Part model, mm, in its own coordinate system. A direction names the side the tool comes from. Coordinates: 2 decimals unless noted, no trailing zeros. Loops run counter-clockwise (first coordinate to the right, second up) from the corner with the lowest first, then second, coordinate; pieces in that order, holes last. Notation, with made-up numbers: M -33.75,47 L 2.25,47 A12 ccw 2.25,57 Z; hole C -8,38 d6. An arc over 180 degrees is marked long. Use a Markdown table: item, result. Add a question column.
1) Band-saw the part on D-D (z = 51). List the corners of the cut face in (x, y).
2) Band-saw the part on C-C (x = 0). List the corners of the cut face in (y, z).
3) Band-saw the part on A-A (x = 22.5). List the corners of the cut face in (y, z).
4) Pin check, flat tips, straight feed: pin 1 Ø15 at (x, y) = (-19.5, -38.5) entering from +Z; pin 2 Ø9.5 at (x, y) = (-22.5, -28) entering from -Z; pin 3 Ø8 at (y, z) = (-9.5, 24) entering from -X; pin 4 Ø12 at (y, z) = (23, 34.5) entering from +X. Stop position of each tip, or through.
5) Pull direction Y, two halves, no side cores. Call faces 5 (the cylindrical face through (21.199, -33.857, 12.084)), 6 (the flat face through (-6, -7, 38)), 7 (the flat face through (0, 13, 19)), 8 (the cylindrical face through (-0.08, 8.05, 62.76)): released by +Y, released by -Y, zero draft, split by the parting line, or undercut.
6) Wall check: probe 1 along Y at (x, z) = (16.5, 5); probe 2 along Y at (x, z) = (22, 9); probe 3 along X at (y, z) = (-27, 29.5). Give the ranges that are in metal, low to high. Write a range as from..to.
7) Band-saw the part on B-B (y = 44). List the corners of the cut face in (x, z), plus the area to 3 significant figures.
8) Tool access for faces 1 (the flat face through (-22, 0, 10)), 2 (the flat face through (22, 0, 10)), 3 (the flat face through (-23, -35, 18)), 4 (the flat face through (1, -44, 3)): list every direction of +Z, -Z, +X, -X, +Y, -Y with a clear straight run to the whole face (end or side of a thin tool).
Solid Edge part; units mm, degrees
sketch "Sketch1" plane through (0, 0, 0) normal (1, 0, 0) x (0, 1, 0)
  line L0 (0, 0) -> (-56, 0)
  line L1 (-56, 0) -> (-56, 18)
  line L2 (-56, 18) -> (0, 18)
  line L3 (0, 0) -> (0, 18)
extrude "Protrusion1" add sketch "Sketch1" along normal mid plane 75
sketch "Sketch2" plane through (37.5, -28, 9) normal (1, 0, 0) x (0, 1, 0)
  line L0 (-16, -9) -> (-16, -3)
  line L1 (-16, -3) -> (16, -3)
  line L2 (16, -3) -> (16, -9)
  line L3 (16, -9) -> (-16, -9)
extrude "ExtrudedCutout_1" cut sketch "Sketch2" against normal blind 100.4669
sketch "Sketch3" plane through (21.75, -28, 18) normal (0, 0, 1) x (1, 0, 0)
  circle A0 centre (0.75, 0) radius 6
  circle A1 centre (-44.25, 0) radius 6
extrude "ExtrudedCutout_2" cut sketch "Sketch3" against normal blind 51.1698
sketch "Sketch4" plane through (0, 0, 0) normal (1, 0, 0) x (0, 1, 0)
  line L0 (8, 63) -> (-56, 18)
  line L1 (-56, 18) -> (0, 18)
  line L2 (0, 0) -> (0, 18)
  line L3 (26, 38) -> (0, 0)
  line L4 (44, 38) -> (26, 38)
  line L5 (44, 38) -> (44, 63)
  line L6 (44, 63) -> (8, 63)
extrude "Protrusion_2" add sketch "Sketch4" along normal mid plane 12
sketch "Sketch5" plane through (0, 26, 63) normal (0, 0, 1) x (0, 1, 0)
  circle A0 centre (18, 0) radius 18
  circle A1 centre (18, 0) radius 11
extrude "Protrusion_3" add sketch "Sketch5" against normal blind 25
sketch "Sketch6" plane through (0, 26, 63) normal (0, 0, 1) x (0, 1, 0)
  circle A0 centre (18, 0) radius 11
extrude "Cutout_3" cut sketch "Sketch6" against normal blind 55.1556
fillet "Round_1" radius 5 3 edges at (0, 8, 63) (6, 27.0294, 50.5) (-6, 27.0294, 50.5)
fillet "Round1" radius 2 2 edges at (6, -28, 18) (-6, -28, 18)
Entries:
| question | item | result |
|---|---|---|
| 1 | outline | M -8.61,28.19 A5 cw -6,23.8 L -6,-9.07 L 6,-9.07 L 6,23.8 A5 cw 8.61,28.19 A18 ccw long Z; hole C 0,44 d22 |
| 2 | outline | M -56,0 L -44,0 L -44,6 L -12,6 L -12,0 L 0,0 L 26,38 L 33,38 L 33,63 L 9.58,63 A5 ccw 6.71,62.09 L -56,18 Z; M 55,38 L 62,38 L 62,63 L 55,63 Z |
| 3 | outline | M -56,0 L -44,0 L -44,6 L -34,6 L -34,18 L -56,18 Z; M -22,6 L -12,6 L -12,0 L 0,0 L 0,18 L -22,18 Z |
| 4 | pin 1 | z = 18 |
| 4 | pin 2 | through |
| 4 | pin 3 | x = -6 |
| 4 | pin 4 | x = 8.1 |
| 5 | face 5 | undercut |
| 5 | face 6 | zero draft |
| 5 | face 7 | released by +Y |
| 5 | face 8 | released by -Y |
| 6 | probe 1 | -56..-44, -12..0 |
| 6 | probe 2 | -56..-33.98, -22.02..0 |
| 6 | probe 3 | -6..6 |
| 7 | outline | M -18,38 L -11,38 L -11,63 L -18,63 Z; M 11,38 L 18,38 L 18,63 L 11,63 Z |
| 7 | area | 350 mm2 |
| 8 | face 1 | +Z, -Z, -X, +Y |
| 8 | face 2 | +Z, -Z, +X, +Y |
| 8 | face 3 | +Z, -X, +Y, -Y |
| 8 | face 4 | -Z, +X, -X |
